Autodesk Inventor part; units mm, degrees
ref_plane "YZ Plane" through (0, 0, 0) normal (1, 0, 0) x (0, 1, 0)
ref_plane "XZ Plane" through (0, 0, 0) normal (0, 1, 0) x (-1, 0, 0)
ref_plane "XY Plane" through (0, 0, 0) normal (0, 0, 1) x (1, 0, 0)
sketch "Esboço1" plane through (0, 0, 0) normal (0, 0, 1) x (1, 0, 0)
  circle A0 centre (0, 0) radius 5
  line L0 (0, 0) -> (0, 22.7) construction
  line L1 (-10, 0) -> (-10, 22.7)
  line L2 (10, 22.7) -> (10, 0)
  arc A1 (-10, 0) -> (10, 0) centre (0, 0) ccw
  arc A2 (10, 22.7) -> (-10, 22.7) centre (0, 22.7) ccw
  line L3 (-25.4, 12.7) -> (25.4, 12.7)
  line L4 (25.4, 12.7) -> (25.4, 32.7)
  line L5 (25.4, 32.7) -> (-25.4, 32.7)
  line L6 (-25.4, 32.7) -> (-25.4, 12.7)
  line L7 (-25.4, 12.7) -> (25.4, 32.7) construction
  line L8 (25.4, 12.7) -> (-25.4, 32.7) construction
  circle A3 centre (0, 20) radius 2.5
  line L9 (25.4, 12.7) -> (-25.4, 12.7)
  line L10 (-25.4, 12.7) -> (-25.4, 27.3)
  line L11 (-25.4, 27.3) -> (25.4, 27.3)
  line L12 (25.4, 27.3) -> (25.4, 12.7)
  line L13 (25.4, 12.7) -> (-25.4, 27.3) construction
  line L14 (-25.4, 12.7) -> (25.4, 27.3) construction
  circle A4 centre (12.7, 20) radius 2.5
  circle A5 centre (-12.7, 20) radius 2.5
  line L15 (18, 12.7) -> (-18, 12.7)
  line L16 (-18, 12.7) -> (-18, 27.3)
  line L17 (-18, 27.3) -> (18, 27.3)
  line L18 (18, 27.3) -> (18, 12.7)
  line L19 (18, 12.7) -> (-18, 27.3) construction
  line L20 (-18, 12.7) -> (18, 27.3) construction
  point P0 (0, 11.35)
  point P1 (25.4, 22.7)
  point P2 (-10, 12.7)
  point P3 (10, 12.7)
  dimension "d0" = 10
  dimension "d1" = 5
  dimension "d2" = 25.4
  dimension "d3" = 5
  dimension "d4" = 12.7
  dimension "d5" = 7.3
  dimension "d6" = 20
  dimension "d9" = 12.7
  dimension "d14" = 18
extrude "Extrusão1" add sketch "Esboço1" along normal blind 4 contours L1 L3 L2 A1 | L3 L16 L11 A2 L1 | L1 A2 L11 L2 L3 | L2 A2 L11 L18 L3
properties part number "Suporte Coletor - Intake"
Geometry check sheet. Reference: the model listing, model coordinates, mm. A direction names the side the tool comes from. Give positions to 0.01 mm unless a question says otherwise; leave off trailing zeros. Loops run counter-clockwise (first coordinate to the right, second up) from the corner with the lowest first, then second, coordinate; pieces in that order, holes last. Notation, with made-up numbers: (10, 28) - (33, 28) arc R18 ccw to (33, 33) - close; hole circle Ø11 at (64.25, 57). An arc over 180 degrees is marked (long way). Use CSV: the item, a comma, the result in double quotes. Start each with the question number.
Q1. Go/stop test with flat-tipped pins: pin 1 Ø2 at (y, z) = (4.5, 3) entering from -X; pin 2 Ø2 at (x, z) = (14.5, 2) entering from -Y; pin 3 Ø2 at (y, z) = (6, 1.5) entering from +X. Record where each tip stops, or that it passes through.
Q2. Scan lines: probe 1 along Y at (x, z) = (0, 3.05); probe 2 along Y at (x, z) = (-12.7, 2); probe 3 along X at (y, z) = (20.5, 1.9). Record each from-to range of solid material in increasing order. Write a range as from..to.
Q3. Access from +Z, -Z, +X, -X, +Y, -Y to the whole of each face (thin tool, end or side, straight path). Record for faces 5 (the face through (0, 13, 0)), 6 (the face through (-10, 6, 2)), 7 (the face through (10, 6, 2)).
Q4. Section check B-B, the plane y = 21.5. Record the cut outline in (x, z).
Q5. Release check for a two-part mould opening along X. For faces 1 (the face through (1.34, 17.89, 1.97)), 2 (the face through (0, -10, 2)), 3 (the face through (-13.03, 17.52, 1.97)), 4 (the face through (0, 27.3, 2)) record: +X half, -X half, draft (parallel to the pull), parting line (faces both ways), or undercut.
Q6. Section check D-D, the plane x = 0. Record the cut outline in (y, z), and give its area (3 significant figures).
Q7. Section check A-A, the plane x = 12.7. Record the cut outline in (y, z).
Q8. Section check C-C, the plane z = 0.9. Record the cut outline in (x, y), and give its area (3 significant figures).
Findings below:
1,pin 1,"stops at x = -10"
1,pin 2,"stops at y = 12.7"
1,pin 3,"stops at x = 10"
2,probe 1,"y = -10..-5, 5..17.5, 22.5..27.3"
2,probe 2,"y = 12.7..17.5, 22.5..27.3"
2,probe 3,"x = -18..-15.15, -10.25..-2.45, 2.45..10.25, 15.15..18"
3,face 5,"-Z, +X, -X, +Y, -Y"
3,face 6,"+Z, -Z, -X, -Y"
3,face 7,"+Z, -Z, +X, -Y"
4,outline,"(-18, 0) - (-14.7, 0) - (-14.7, 4) - (-18, 4) - close; (-10.7, 0) - (-2, 0) - (-2, 4) - (-10.7, 4) - close; (2, 0) - (10.7, 0) - (10.7, 4) - (2, 4) - close; (14.7, 0) - (18, 0) - (18, 4) - (14.7, 4) - close"
5,face 1,"undercut"
5,face 2,"parting line"
5,face 3,"undercut"
5,face 4,"draft"
6,outline,"(-10, 0) - (-5, 0) - (-5, 4) - (-10, 4) - close; (5, 0) - (17.5, 0) - (17.5, 4) - (5, 4) - close; (22.5, 0) - (27.3, 0) - (27.3, 4) - (22.5, 4) - close"
6,area,"89.2 mm^2"
7,outline,"(12.7, 0) - (17.5, 0) - (17.5, 4) - (12.7, 4) - close; (22.5, 0) - (27.3, 0) - (27.3, 4) - (22.5, 4) - close"
8,outline,"(-18, 12.7) - (-10, 12.7) - (-10, 0) arc R10 ccw to (10, 0) - (10, 12.7) - (18, 12.7) - (18, 27.3) - (-18, 27.3) - close; hole circle Ø5 at (-12.7, 20); hole circle Ø10 at (0, 0); hole circle Ø5 at (0, 20); hole circle Ø5 at (12.7, 20)"
8,area,"799 mm^2"
